```python
from build123d import *

# Parameters (mm, degrees)
F0_R     = 12.7
F1_DEPTH = 25.4
F2_R     = 12.7
F3_DEPTH = 25.4
F4_DEPTH = 25.4
F5_R     = 12.7


with BuildPart() as f1:
    # F0 (on Front) → F1 (new body)
    with BuildSketch(Plane.XZ):
        with BuildLine():
            Line((101.463508, -37.634854), (13.885502, 21.179284))
            ThreePointArc((13.885502, 21.179284), (-12.263588, 22.485844), (-25.675108, 0))
            Line((-25.675108, 0), (-25.489152, -50.79966))
            Line((-25.489152, -50.79966), (101.509997, -50.334769))
            Line((101.509997, -50.334769), (101.463508, -37.634854))
        make_face()
        with Locations((-0.306273, 0.13584)):
            Circle(F0_R, mode=Mode.SUBTRACT)
    extrude(amount=F1_DEPTH)

    # F2 (on face) → F3 (join)
    with BuildSketch(Plane.XZ.offset(25.4)):
        with BuildLine():
            Line((25.4, -37.634854), (25.4, 0))
            ThreePointArc((25.4, 0), (22.860903, 11.069738), (15.751252, 19.926316))
            Line((15.751252, 19.926316), (13.885502, 21.179284))
            ThreePointArc((13.885502, 21.179284), (11.033245, 22.836709), (7.990239, 24.110497))
            ThreePointArc((7.990239, 24.110497), (-15.064639, 20.743276), (-25.675108, 0))
            Line((-25.675108, 0), (-25.535641, -38.099745))
            Line((-25.535641, -38.099745), (-25.489152, -50.79966))
            Line((-25.489152, -50.79966), (101.463508, -50.334939))
            Line((101.463508, -50.334939), (101.463508, -37.634854))
            Line((101.463508, -37.634854), (25.4, -37.634854))
        make_face()
        with Locations((-0.306273, 0.13584)):
            Circle(F2_R, mode=Mode.SUBTRACT)
    extrude(amount=F3_DEPTH)

    # F2 (on face) → F4 (join)
    with BuildSketch(Plane.XZ.offset(25.4)):
        with BuildLine():
            Line((25.4, -37.634854), (25.4, 0))
            ThreePointArc((25.4, 0), (22.860903, 11.069738), (15.751252, 19.926316))
            Line((15.751252, 19.926316), (13.885502, 21.179284))
            ThreePointArc((13.885502, 21.179284), (11.033245, 22.836709), (7.990239, 24.110497))
            ThreePointArc((7.990239, 24.110497), (-15.064639, 20.743276), (-25.675108, 0))
            Line((-25.675108, 0), (-25.535641, -38.099745))
            Line((-25.535641, -38.099745), (-25.489152, -50.79966))
            Line((-25.489152, -50.79966), (101.463508, -50.334939))
            Line((101.463508, -50.334939), (101.463508, -37.634854))
            Line((101.463508, -37.634854), (25.4, -37.634854))
        make_face()
        with Locations((-0.306273, 0.13584)):
            Circle(F2_R, mode=Mode.SUBTRACT)
    extrude(amount=F4_DEPTH)

    # F5
    f5_edges = [f1.edges().sort_by_distance(p)[0] for p in [
        (101.463508, -50.8, -43.984897),
    ]]
    fillet(f5_edges, radius=F5_R)


solid = f1.part
```
Verification items for the finished model (mm, model axes). A direction names the side the tool comes from. Coordinates: 2 decimals unless noted, no trailing zeros. Write each loop counter-clockwise with the first axis right and the second up, starting at its lowest first coordinate (ties: lowest second). Pieces come first, ordered by that corner, then holes. Notation, with made-up numbers: (-6.5, 3.5) - (29.5, 3.5) arc R24 ccw to (29.5, 27.5) - close; hole circle Ø2 at (72.5, 52). An arc over 180 degrees is marked (long way). One line per question, with ' | ' between items. Start each with the question number.
1. Gauge pin test, flat ends, axial feed: P1, Ø10, axis at x = 6, y = -45.5, coming from the -Z side; P2, Ø5, axis at y = -36.5, z = -28, coming from the -X side; P3, Ø10, axis at y = -39, z = -20, coming from the +X side. Record the tip position at first contact, or that the pin passes through.
2. Access from +Z, -Z, +X, -X, +Y, -Y to the whole of each face (thin tool, end or side, straight path). Record for faces 1 (the flat face through (5, -50.8, -21)), 2 (the cylindrical face through (22.93, -37.92, 10.93)).
3. Section check D-D (z = -7). Enter the section's corners in (x, y), plus the area to 3 significant figures.
4. Section check C-C (x = 19). Enter the section's corners in (y, z).
5. Material ranges on line 1 along Y through (x, z) = (25, 9); line 2 along X through (y, z) = (-25, -45.5); line 3 along X through (y, z) = (-42.5, -6.5), recorded low to high.
6. Draft check along X on faces 3 (the flat face through (101.464, -32, -44)), 4 (the flat face through (64, -38, -37.635)), 5 (the cylindrical face through (11.807, -25.044, 3.951)). Enter one of: released by +X, released by -X, zero draft, split by the parting line, or undercut.
7. Section check A-A (z = 8). Enter the section's corners in (x, y).
8. Section check B-B (y = -39.5). Enter the section's corners in (x, z).
Computed values:
1) P1: z = -50.7 | P2: x = -25.58 | P3: x = 25.4
2) face 1: +Z, -Z, +X, -X, -Y | face 2: +Z, +X, -Y
3) outline: (-25.65, -50.8) - (-10.81, -50.8) - (-10.81, 0) - (-25.65, 0) - close; (10.2, -50.8) - (25.4, -50.8) - (25.4, -25.4) - (55.85, -25.4) - (55.85, 0) - (10.2, 0) - close | area: 2,300 mm²
4) outline: (-50.8, -50.64) - (0, -50.64) - (0, 17.74) - (-25.4, 17.74) - (-25.4, 16.86) - (-50.8, 16.86) - close
5) line 1: -25.4 to 0 | line 2: -25.51 to 101.49 | line 3: -25.65 to -11.13, 10.52 to 25.4
6) face 3: released by +X | face 4: zero draft | face 5: undercut
7) outline: (-24.41, -50.8) - (-10.28, -50.8) - (-10.28, 0) - (-24.41, 0) - close; (9.67, -50.8) - (24.11, -50.8) - (24.11, -25.4) - (33.51, -25.4) - (33.51, 0) - (9.67, 0) - close
8) outline: (-25.68, 0) - (-25.49, -50.8) - (101.39, -50.34) - (101.39, -37.63) - (25.4, -37.63) - (25.4, 0) arc R25.4 ccw to (15.75, 19.93) - (13.89, 21.18) arc R25.4 ccw to (7.99, 24.11) arc R25.4 ccw to start; hole circle Ø25.4 at (-0.31, 0.14)
